For this review, take the finished solid that the model builds, in its own axes (mm). A direction names the side the tool comes from. Coordinates: 2 decimals unless noted, no trailing zeros. Write each loop counter-clockwise with the first axis right and the second up, starting at its lowest first coordinate (ties: lowest second). Pieces come first, ordered by that corner, then holes. Notation, with made-up numbers: M 75,80 L 84,80 A18 cw 84,90 Z; hole C 56,13 d8. An arc over 180 degrees is marked long. One line per question, with ' | ' between items.
from build123d import *

# Parameters (mm, degrees)
SKETCH1_R           = 2.75
BOSS_EXTRUDE1_DEPTH = 4


with BuildPart() as part:
    # Sketch1 → Boss-Extrude1 (new body)
    with BuildSketch(Plane.XY):
        with BuildLine():
            Line((-60, 35), (-53.828555675, 70))
            Line((-53.828555675, 70), (-33.828555675, 70))
            Line((-33.828555675, 70), (-37.930541604, 46.736481777))
            ThreePointArc((-37.930541604, 46.736481777), (-35.742908505, 38.572123903), (-28.082464074, 35))
            Line((-28.082464074, 35), (30, 35))
            ThreePointArc((30, 35), (37.071067812, 37.928932188), (40, 45))
            Line((40, 45), (40, 70))
            Line((40, 70), (60, 70))
            Line((60, 70), (60, 35))
            Line((60, 35), (60, -35))
            Line((60, -35), (-60, -35))
            Line((-60, -35), (-60, 35))
        make_face()
        with Locations((-50, 25)):
            Circle(SKETCH1_R, mode=Mode.SUBTRACT)
        with Locations((-50, -25)):
            Circle(SKETCH1_R, mode=Mode.SUBTRACT)
        with Locations((50, 25)):
            Circle(SKETCH1_R, mode=Mode.SUBTRACT)
        with Locations((50, -25)):
            Circle(SKETCH1_R, mode=Mode.SUBTRACT)
        with BuildLine():
            Line((-49.341825482, 57.25), (-41.841825482, 57.25))
            ThreePointArc((-41.841825482, 57.25), (-39.091825482, 60), (-41.841825482, 62.75))
            Line((-41.841825482, 62.75), (-49.341825482, 62.75))
            ThreePointArc((-49.341825482, 62.75), (-52.091825482, 60), (-49.341825482, 57.25))
        make_face(mode=Mode.SUBTRACT)
        with BuildLine():
            Line((-27.5, -16.25), (27.5, -16.25))
            ThreePointArc((27.5, -16.25), (43.75, 0), (27.5, 16.25))
            Line((27.5, 16.25), (-27.5, 16.25))
            ThreePointArc((-27.5, 16.25), (-43.75, 0), (-27.5, -16.25))
        make_face(mode=Mode.SUBTRACT)
        with BuildLine():
            Line((46.25, 57.25), (53.75, 57.25))
            ThreePointArc((53.75, 57.25), (56.5, 60), (53.75, 62.75))
            Line((53.75, 62.75), (46.25, 62.75))
            ThreePointArc((46.25, 62.75), (43.5, 60), (46.25, 57.25))
        make_face(mode=Mode.SUBTRACT)
    extrude(amount=BOSS_EXTRUDE1_DEPTH)


solid = part.part
1. Draft analysis for pull direction Y (two halves, no side actions). For faces 1 (the flat face through (0, 16.25, 2)), 2 (the flat face through (-44, 70, 2)), 3 (the flat face through (40, 57, 2)), 4 (the cylindrical face through (43.5, 60.1, 2)), state which applies: pulls with the +Y half, pulls with the -Y half, needs draft (parallel to the pull), parting line crosses it, or undercut.
Computed values:
face 1: undercut | face 2: pulls with the +Y half | face 3: needs draft | face 4: undercut
2. Clearance check with flat-ended pins moving along their axes: P1, Ø2, axis at x = 13, z = 1, coming from the +Y side; P2, Ø1.2, axis at y = 60, z = 1.5, coming from the -X side. State where each tip first meets the part, or that it passes through.
Computed values:
P1: stops at y = 35 | P2: stops at x = -55.7
3. For line 1 along Y through (x, z) = (50, 1.15); line 2 along Y through (x, z) = (-28, 0.2); line 3 along X through (y, z) = (59, 2.3), list the stretches that pass through material, from the lowest coordinate up.
Computed values:
line 1: y = -35 to -27.75, -22.25 to 22.25, 27.75 to 57.25, 62.75 to 70 | line 2: y = -35 to -16.24, 16.24 to 35 | line 3: x = -55.77 to -51.9, -39.28 to -35.77, 40 to 43.69, 56.31 to 60
4. Take a section at B-B on x = 23. State the section outline as (y, z) points, plus the area to 3 significant figures.
Computed values:
outline: M -35,0 L -16.25,0 L -16.25,4 L -35,4 Z; M 16.25,0 L 35,0 L 35,4 L 16.25,4 Z | area: 150 mm2
5. Take a section at C-C on y = 25. State the section outline as (x, z) points, plus the area to 3 significant figures.
Computed values:
outline: M -60,0 L -52.75,0 L -52.75,4 L -60,4 Z; M -47.25,0 L 47.25,0 L 47.25,4 L -47.25,4 Z; M 52.75,0 L 60,0 L 60,4 L 52.75,4 Z | area: 436 mm2
6. Machinability: for faces 5 (the cylindrical face through (36.99, 37.85, 1.97)), 6 (the flat face through (1, 18, 0)), 7 (the cylindrical face through (-52.09, 60.06, 1.97)), which of the approach directions +Z, -Z, +X, -X, +Y, -Y give a long, thin tool a straight path to every point of the face, cutting with its end or side? Answer none if there is none.
Computed values:
face 5: +Z, -Z, +Y | face 6: -Z, +X, -X, +Y, -Y | face 7: +Z, -Z
7. Take a section at D-D on z = 1.7. State the section outline as (x, y) points, plus the area to 3 significant figures.
Computed values:
outline: M -60,-35 L 60,-35 L 60,70 L 40,70 L 40,45 A10 cw 30,35 L -28.08,35 A10 cw -37.93,46.74 L -33.83,70 L -53.83,70 L -60,35 Z; hole C -50,-25 d5.5; hole C -50,25 d5.5; hole M -49.34,57.25 L -41.84,57.25 A2.75 ccw -41.84,62.75 L -49.34,62.75 A2.75 ccw Z; hole M -27.5,-16.25 L 27.5,-16.25 A16.25 ccw 27.5,16.25 L -27.5,16.25 A16.25 ccw Z; hole M 46.25,57.25 L 53.75,57.25 A2.75 ccw 53.75,62.75 L 46.25,62.75 A2.75 ccw Z; hole C 50,-25 d5.5; hole C 50,25 d5.5 | area: 7,010 mm2
8. Take a section at A-A on y = 0. State the section outline as (x, z) points, plus the area to 3 significant figures.
Computed values:
outline: M -60,0 L -43.75,0 L -43.75,4 L -60,4 Z; M 43.75,0 L 60,0 L 60,4 L 43.75,4 Z | area: 130 mm2
